Design review of the part built by this model. Coordinates are the model's own, in mm. Face numbers are marked on the shaded views. Coordinates: 2 decimals unless noted, no trailing zeros. Order: outer loops, then holes, each group sorted by start corner. A loop starts at its lowest first (then second) coordinate and runs counter-clockwise, first axis right, second up. Notation, with made-up numbers: (2.5, 84.5) - (23.5, 84.5) arc R24 ccw to (23.5, 113.5) - close; hole circle Ø9 at (4, 50.5). An arc over 180 degrees is marked (long way). Write each question's results on one line, items separated by ' | '. Start each with the question number.
Autodesk Fusion 360 part; units mm, degrees
sketch "Esquisse1" plane through (0, 0, 0) normal (0, 1, 0) x (1, 0, 0)
  circle A0 centre (0, 0) radius 35
  circle A1 centre (0, 0) radius 50
  line L0 (42.5, 0) -> (21.25, 36.8061) construction
  line L1 (21.25, 36.8061) -> (-21.25, 36.8061) construction
  line L2 (-21.25, 36.8061) -> (-42.5, 0) construction
  line L3 (-42.5, 0) -> (-21.25, -36.8061) construction
  line L4 (-21.25, -36.8061) -> (21.25, -36.8061) construction
  line L5 (21.25, -36.8061) -> (42.5, 0) construction
  circle A2 centre (0, 0) radius 42.5 construction
  line L6 (50, 0) -> (-50, 0)
  line L7 (0, -50) -> (0, 50)
  circle A3 centre (21.25, -36.8061) radius 1.6
  circle A4 centre (-21.25, -36.8061) radius 1.6
  circle A5 centre (-42.5, 0) radius 1.6
  circle A6 centre (-21.25, 36.8061) radius 1.6
  circle A7 centre (21.25, 36.8061) radius 1.6
  circle A8 centre (42.5, 0) radius 1.6
  dimension "d1" = 70
  dimension "d2" = 15
  dimension "d5" = 7.5
  dimension "d6" = 3.2
extrude "Extrusion1" add sketch "Esquisse1" along normal blind 10 contours A0 A1 L6 L7 A8 | A0 A1 L6 L7 A8 | A0 A1 L6 L7 A5 | A0 A1 L6 L7 A5
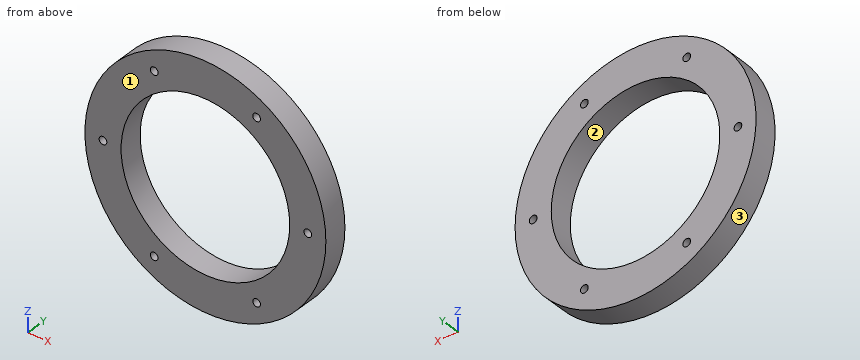
(1) To check wall thickness, follow line 1 along X through (y, z) = (3.75, 0); line 2 along Z through (x, y) = (-22, 5.25); line 3 along Z through (x, y) = (21.25, 2.5). State the ranges of each line that lie inside material, in increasing order. Write a range as [from, to].
(2) Clearance check with flat-ended pins moving along their axes: pin 1 (1.5 mm diameter, centred on y = 6.5, z = -21, fed in from -X); pin 2 (2.5 mm diameter, centred on x = 42.5, z = 0, fed in from +Y); pin 3 (4 mm diameter, centred on y = 1.5, z = 13, fed in from +X) (3 decimals). State where each tip first meets the part, or that it passes through.
(3) Take a section at C-C (x = -21.25). State the section outline as (y, z) points.
(4) Take a section at B-B (z = 0). State the section outline as (x, y) points.
(5) Mouldability with a two-part tool opening along Z and no side actions: class the marked faces 1, 2 and 3 as +Z half, -Z half, draft (parallel to the pull), parting line (faces both ways), or undercut.
(6) Take a section at A-A (x = 0). State the section outline as (y, z) points, plus the area to 3 significant figures.
(7) Take a section at D-D (z = -30.5). State the section outline as (x, y) points, plus the area to 3 significant figures.
Worked out:
1) line 1: [-50, -44.1], [-40.9, -35], [35, 40.9], [44.1, 50] | line 2: [-44.9, -38.22], [-35.39, -27.22], [27.22, 35.39], [38.22, 44.9] | line 3: [-45.26, -38.41], [-35.21, -27.81], [27.81, 35.21], [38.41, 45.26]
2) pin 1: x = -45.72 | pin 2: through | pin 3: x = 48.775
3) outline: (0, -45.26) - (10, -45.26) - (10, -38.41) - (0, -38.41) - close; (0, -35.21) - (10, -35.21) - (10, -27.81) - (0, -27.81) - close; (0, 27.81) - (10, 27.81) - (10, 35.21) - (0, 35.21) - close; (0, 38.41) - (10, 38.41) - (10, 45.26) - (0, 45.26) - close
4) outline: (-50, 0) - (-44.1, 0) - (-44.1, 10) - (-50, 10) - close; (-40.9, 0) - (-35, 0) - (-35, 10) - (-40.9, 10) - close; (35, 0) - (40.9, 0) - (40.9, 10) - (35, 10) - close; (44.1, 0) - (50, 0) - (50, 10) - (44.1, 10) - close
5) face 1: draft | face 2: undercut | face 3: parting line
6) outline: (0, -50) - (10, -50) - (10, -35) - (0, -35) - close; (0, 35) - (10, 35) - (10, 50) - (0, 50) - close | area: 300 mm^2
7) outline: (-39.62, 0) - (-17.17, 0) - (-17.17, 10) - (-39.62, 10) - close; (17.17, 0) - (39.62, 0) - (39.62, 10) - (17.17, 10) - close | area: 449 mm^2
